The listing builds one solid part. Answer for the finished solid, in the listing's coordinates (mm). Round coordinates to 2 decimals unless told otherwise and drop trailing zeros. Write each loop counter-clockwise with the first axis right and the second up, starting at its lowest first coordinate (ties: lowest second). Pieces come first, ordered by that corner, then holes.
Item 1: Find section A-A on z = 1.3. Give the number of separate pieces and of enclosed holes in the cut face, then the cut area to 3 significant figures.
Item 2: Find section B-B on x = 42. Give the vertices of the cut face in (y, z) (3 decimals).
Item 3: Find section C-C on y = 212. Give the vertices of the cut face in (x, z) (3 decimals).
Item 4: Each of these flat-tipped pins is pushed along its axis until it touches: pin 1 (4.5 mm diameter, centred on x = 182.26, y = 285.75, fed in from +Z); pin 2 (1.5 mm diameter, centred on y = 57, z = 1.5, fed in from +X); pin 3 (1 mm diameter, centred on x = 189.5, z = 1, fed in from -Y). Where does it stop, or does it pass through?
Item 5: Find the intervals of material crossed by probe 1 along X at (y, z) = (23.5, 1.75); probe 2 along Y at (x, z) = (173.5, 1.7); probe 3 along Y at (x, z) = (130.5, 0.1), in increasing order.
```python
from build123d import *

# Parameters (mm, degrees)
BOSS_EXTRUDE1_DEPTH = 3.175
SKETCH2_R           = 2.5527
SKETCH2_R_2         = 2.522358926
CUT_EXTRUDE1_DEPTH  = 351.604295129
SKETCH3_R           = 2.5527
CUT_EXTRUDE2_DEPTH  = 351.604295129


with BuildPart() as part:
    # Sketch1 → Boss-Extrude1 (new body)
    with BuildSketch(Plane.XY):
        Polygon((0, 0), (0, 38.1), (170.441996978, 290.790652115), (195.841996978, 290.790652115), (195.841996978, 245.368044206), (170.441996978, 245.368044206), (30.637935892, 38.1), (30.637935892, 0), align=None)
    extrude(amount=BOSS_EXTRUDE1_DEPTH)

    # Sketch2 → Cut-Extrude1 (cut, through all)
    with BuildSketch(Plane.XY.offset(3.175)):
        with Locations((182.257063518, 285.750000017)):
            Circle(SKETCH2_R)
        with Locations((182.257063518, 273.050000017)):
            Circle(SKETCH2_R)
        with Locations((23.380063476, 12.7)):
            Circle(SKETCH2_R_2)
        with Locations((10.680063476, 12.7)):
            Circle(SKETCH2_R)
        with Locations((182.257063518, 260.350000017)):
            Circle(SKETCH2_R)
    extrude(amount=-CUT_EXTRUDE1_DEPTH, mode=Mode.SUBTRACT)

    # Sketch3 → Cut-Extrude2 (cut, through all)
    with BuildSketch(Plane.XY.offset(3.175)):
        with Locations((104.936582102, 182.319228816)):
            Circle(SKETCH3_R)
        with Locations((129.668859022, 196.275033285)):
            Circle(SKETCH3_R)
        with Locations((119.14008185, 203.376783159)):
            Circle(SKETCH3_R)
        with Locations((115.465359274, 175.217478942)):
            Circle(SKETCH3_R)
        with Locations((50.353519505, 101.396510668)):
            Circle(SKETCH3_R)
        with Locations((64.557019253, 122.454065011)):
            Circle(SKETCH3_R)
        with Locations((75.085796425, 115.352315137)):
            Circle(SKETCH3_R)
        with Locations((60.882296677, 94.294760794)):
            Circle(SKETCH3_R)
    extrude(amount=-CUT_EXTRUDE2_DEPTH, mode=Mode.SUBTRACT)


solid = part.part
```
Check values:
1. separate pieces: 1
1. enclosed holes: 13
1. area: 9,100 mm2
2. outline: (54.945, 0) - (100.368, 0) - (100.368, 3.175) - (54.945, 3.175) - close
3. outline: (117.297, 0) - (147.935, 0) - (147.935, 3.175) - (117.297, 3.175) - close
4. pin 1: passes through
4. pin 2: stops at x = 43.89
4. pin 3: stops at y = 245.37
5. probe 1: x = 0 to 30.64
5. probe 2: y = 245.37 to 290.79
5. probe 3: y = 186.15 to 193.86, 198.69 to 231.57
